Here's how the part is built. I have some questions about the finished solid (model axes, mm). Face numbers are marked on the shaded views. A direction names the side the tool comes from. Give positions to 0.01 mm unless a question says otherwise; leave off trailing zeros. Order: outer loops, then holes, each group sorted by start corner. A loop starts at its lowest first (then second) coordinate and runs counter-clockwise, first axis right, second up. Notation, with made-up numbers: M 43,75.5 L 90,75.5 A6 ccw 90,84.5 Z; hole C 86.5,-4.5 d3. An arc over 180 degrees is marked long. One line per item, written item: value. Start each with the question number.
from build123d import *

# Parameters (mm, degrees)
F0_W          = 62
F0_H          = 90
F1_DEPTH      = 3
F2_W          = 62
F2_H          = 26
F3_DEPTH      = 10
F4_R          = 9.5
F5_DEPTH      = 29
F6_R          = 6
F7_DEPTH      = 31.001
F7_DEPTH_BACK = 31.001
F8_R          = 12.5
F8_R_2        = 1.55
F9_DEPTH      = 13.001
F18_DEPTH     = 2
F19_W         = 8
F19_H         = 25.5
F20_DEPTH     = 10
F21_W         = 8
F21_H         = 2.25
F22_DEPTH     = 10
F23_W         = 8
F23_H         = 4
F24_DEPTH     = 10
F25_SIZE      = 1


with BuildPart() as f1:
    # F0 (on Top) → F1 (new body)
    with BuildSketch(Plane.XY):
        Rectangle(F0_W, F0_H)
    extrude(amount=F1_DEPTH)

    # F2 (on face) → F3 (join)
    with BuildSketch(Plane(origin=(0, 0, 0), x_dir=(1, 0, 0), z_dir=(0, 0, -1))):
        with Locations((0, 32)):
            Rectangle(F2_W, F2_H)
        with Locations((0, -32)):
            Rectangle(F2_W, F2_H)
    extrude(amount=F3_DEPTH)

    # F4 (on Right) → F5 (cut, symmetric)
    with BuildSketch(Plane.YZ):
        with Locations((-32, -10)):
            Circle(F4_R)
        with Locations((32, -10)):
            Circle(F4_R)
    extrude(amount=F5_DEPTH, both=True, mode=Mode.SUBTRACT)

    # F6 (on Right) → F7 (cut, two sides)
    with BuildSketch(Plane.YZ) as f7_sk:
        with Locations((-32, -10)):
            Circle(F6_R)
        with Locations((32, -10)):
            Circle(F6_R)
    extrude(amount=-F7_DEPTH, mode=Mode.SUBTRACT)
    extrude(f7_sk.sketch, amount=F7_DEPTH_BACK, mode=Mode.SUBTRACT)

    # F8 (on face) → F9 (cut, through all)
    with BuildSketch(Plane.XY.offset(3)):
        with Locations((0, -7)):
            Circle(F8_R)
        with Locations((-17.5, -7)):
            Circle(F8_R_2)
        with Locations((17.5, -7)):
            Circle(F8_R_2)
    extrude(amount=-F9_DEPTH, mode=Mode.SUBTRACT)

    # F11 (on offset) + F13 (on offset) + F15 (on offset) + F17 (on offset) → F18 (cut, symmetric)
    with BuildSketch(Plane.YZ.offset(23)):
        with BuildLine():
            Line((-44, 3), (-44, -10))
            Line((-44, -10), (-42, -10))
            Line((-42, -10), (-42, -4))
            ThreePointArc((-42, -4), (-40.5355339059, -0.4644660941), (-37, 1))
            Line((-37, 1), (-27, 1))
            ThreePointArc((-27, 1), (-23.4644660941, -0.4644660941), (-22, -4))
            Line((-22, -4), (-22, -10))
            Line((-22, -10), (-20, -10))
            Line((-20, -10), (-20, 3))
            Line((-20, 3), (-44, 3))
        make_face()
        with BuildLine():
            Line((42, -4), (42, -10))
            Line((42, -10), (44, -10))
            Line((44, -10), (44, 3))
            Line((44, 3), (20, 3))
            Line((20, 3), (20, -10))
            Line((20, -10), (22, -10))
            Line((22, -10), (22, -4))
            ThreePointArc((22, -4), (23.4644660941, -0.4644660941), (27, 1))
            Line((27, 1), (37, 1))
            ThreePointArc((37, 1), (40.5355339059, -0.4644660941), (42, -4))
        make_face()
    with BuildSketch(Plane.YZ.offset(6)):
        with BuildLine():
            Line((-44, 3), (-44, -10))
            Line((-44, -10), (-42, -10))
            Line((-42, -10), (-42, -4))
            ThreePointArc((-42, -4), (-40.5355339059, -0.4644660941), (-37, 1))
            Line((-37, 1), (-27, 1))
            ThreePointArc((-27, 1), (-23.4644660941, -0.4644660941), (-22, -4))
            Line((-22, -4), (-22, -10))
            Line((-22, -10), (-20, -10))
            Line((-20, -10), (-20, 3))
            Line((-20, 3), (-44, 3))
        make_face()
        with BuildLine():
            Line((20, -10), (22, -10))
            Line((22, -10), (22, -4))
            ThreePointArc((22, -4), (23.4644660941, -0.4644660941), (27, 1))
            Line((27, 1), (37, 1))
            ThreePointArc((37, 1), (40.5355339059, -0.4644660941), (42, -4))
            Line((42, -4), (42, -10))
            Line((42, -10), (44, -10))
            Line((44, -10), (44, 3))
            Line((44, 3), (20, 3))
            Line((20, 3), (20, -10))
        make_face()
    with BuildSketch(Plane.YZ.offset(-23)):
        with BuildLine():
            Line((-44, 3), (-44, -10))
            Line((-44, -10), (-42, -10))
            Line((-42, -10), (-42, -4))
            ThreePointArc((-42, -4), (-40.5355339059, -0.4644660941), (-37, 1))
            Line((-37, 1), (-27, 1))
            ThreePointArc((-27, 1), (-23.4644660941, -0.4644660941), (-22, -4))
            Line((-22, -4), (-22, -10))
            Line((-22, -10), (-20, -10))
            Line((-20, -10), (-20, 3))
            Line((-20, 3), (-44, 3))
        make_face()
        with BuildLine():
            Line((42, -10), (44, -10))
            Line((44, -10), (44, 3))
            Line((44, 3), (20, 3))
            Line((20, 3), (20, -10))
            Line((20, -10), (22, -10))
            Line((22, -10), (22, -4))
            ThreePointArc((22, -4), (23.4644660941, -0.4644660941), (27, 1))
            Line((27, 1), (37, 1))
            ThreePointArc((37, 1), (40.5355339059, -0.4644660941), (42, -4))
            Line((42, -4), (42, -10))
        make_face()
    with BuildSketch(Plane.YZ.offset(-6)):
        with BuildLine():
            Line((-44, 3), (-44, -10))
            Line((-44, -10), (-42, -10))
            Line((-42, -10), (-42, -4))
            ThreePointArc((-42, -4), (-40.5355339059, -0.4644660941), (-37, 1))
            Line((-37, 1), (-27, 1))
            ThreePointArc((-27, 1), (-23.4644660941, -0.4644660941), (-22, -4))
            Line((-22, -4), (-22, -10))
            Line((-22, -10), (-20, -10))
            Line((-20, -10), (-20, 3))
            Line((-20, 3), (-44, 3))
        make_face()
        with BuildLine():
            Line((42, -4), (42, -10))
            Line((42, -10), (44, -10))
            Line((44, -10), (44, 3))
            Line((44, 3), (20, 3))
            Line((20, 3), (20, -10))
            Line((20, -10), (22, -10))
            Line((22, -10), (22, -4))
            ThreePointArc((22, -4), (23.4644660941, -0.4644660941), (27, 1))
            Line((27, 1), (37, 1))
            ThreePointArc((37, 1), (40.5355339059, -0.4644660941), (42, -4))
        make_face()
    extrude(amount=F18_DEPTH, both=True, mode=Mode.SUBTRACT)

    # F19 (on face) → F20 (join)
    with BuildSketch(Plane(origin=(0, 0, 0), x_dir=(1, 0, 0), z_dir=(0, 0, -1))):
        with Locations((27, 0)):
            Rectangle(F19_W, F19_H)
        with Locations((-27, 0)):
            Rectangle(F19_W, F19_H)
    extrude(amount=F20_DEPTH)

    # F21 (on face) → F22 (cut, through all)
    with BuildSketch(Plane(origin=(0, 0, -10), x_dir=(1, 0, 0), z_dir=(0, 0, -1))):
        with Locations((-27, 7.625)):
            Rectangle(F21_W, F21_H)
        with Locations((27, -7.625)):
            Rectangle(F21_W, F21_H)
    extrude(amount=-F22_DEPTH, mode=Mode.SUBTRACT)

    # F23 (on face) → F24 (join)
    with BuildSketch(Plane(origin=(0, 0, -10), x_dir=(1, 0, 0), z_dir=(0, 0, -1))):
        with Locations((-27, -10.75)):
            Rectangle(F23_W, F23_H)
        with Locations((27, 10.75)):
            Rectangle(F23_W, F23_H)
        with Locations((-27, -4.5)):
            Rectangle(F23_W, F23_H)
        with Locations((27, 4.5)):
            Rectangle(F23_W, F23_H)
    extrude(amount=F24_DEPTH)

    # F25
    f25_edges = [f1.edges().sort_by_distance(p)[0] for p in [
        (-23, -8.75, -5),
        (-23, -6.5, -5),
        (-23, 6.5, -15),
        (-23, 8.75, -15),
        (23, 6.5, -5),
        (23, 8.75, -5),
        (23, -6.5, -15),
        (23, -8.75, -15),
    ]]
    chamfer(f25_edges, length=F25_SIZE)


solid = f1.part
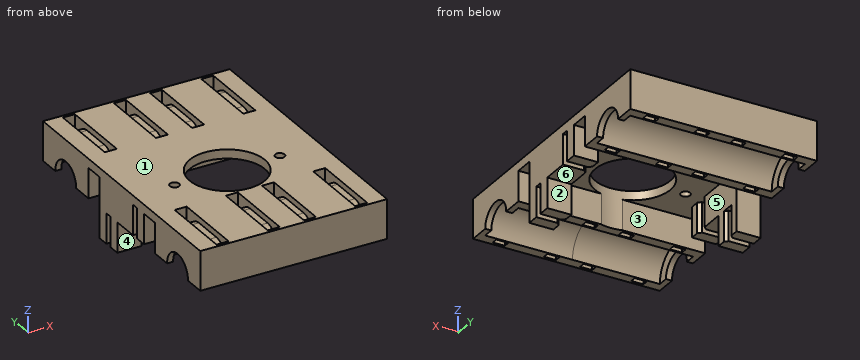
Item 1: Will these pins go through, and if not, where does the flat tip stop? P1, Ø1.5, axis at x = -22, y = 26.5, coming from the -Z side; P2, Ø4, axis at x = 4, y = 17.5, coming from the -Z side; P3, Ø1.2, axis at x = 6, y = -31.5, coming from the +Z side.
Item 2: I want a section at C-C on y = -32. Write out the boundary of the cut face in (x, z), plus the area to 3 significant figures.
Item 3: For the marked faces 4, 5 and 6, which set-ups out of +Z, -Z, +X, -X, +Y, -Y let a thin tool reach every point of the face, with its end or its side?
Item 4: I want a section at A-A on z = -17.5. Write out the boundary of the cut face in (x, y), plus the area to 3 significant figures.
Item 5: I want a section at B-B on x = -17.5. Write out the boundary of the cut face in (y, z), plus the area to 3 significant figures.
Item 6: I want a section at D-D on z = -5.25. Count the separate pieces of the cut face and the enclosed holes in it, plus the area to 3 significant figures.
Item 7: Please list where these lines run through material, in increasing order: probe 1 along X at (y, z) = (40.5, 0.75); probe 2 along X at (y, z) = (11, -1.75); probe 3 along Y at (x, z) = (-13.5, -5.75). Write a range as [from, to].
Item 8: We'd pull the mould along Y, two halves only. Please class the marked faces 1, 2 and 3: +Y half, -Y half, draft (parallel to the pull), parting line (faces both ways), or undercut.
Answer below:
1. P1: stops at z = -2.85
1. P2: stops at z = -10
1. P3: stops at z = 1
2. outline: M -31,-4 L -29,-4 L -29,-0.5 L 29,-0.5 L 29,-4 L 31,-4 L 31,3 L 25,3 L 25,1 L 21,1 L 21,3 L 8,3 L 8,1 L 4,1 L 4,3 L -4,3 L -4,1 L -8,1 L -8,3 L -21,3 L -21,1 L -25,1 L -25,3 L -31,3 Z
2. area: 199 mm²
3. face 4: -Z, +X, -X, -Y
3. face 5: -Z
3. face 6: -Z, +X, +Y
4. outline: M -31,2.5 L -23,2.5 L -23,5.5 L -24,6.5 L -31,6.5 Z; M -31,8.75 L -24,8.75 L -23,9.75 L -23,12.75 L -31,12.75 Z; M 23,-12.75 L 31,-12.75 L 31,-8.75 L 24,-8.75 L 23,-9.75 Z; M 23,-5.5 L 24,-6.5 L 31,-6.5 L 31,-2.5 L 23,-2.5 Z
4. area: 126 mm²
5. outline: M -45,-10 L -41.5,-10 A9.5 cw -22.5,-10 L -19,-10 L -19,0 L -8.55,0 L -8.55,3 L -45,3 Z; M -5.45,0 L 19,0 L 19,-10 L 22.5,-10 A9.5 cw 41.5,-10 L 45,-10 L 45,3 L -5.45,3 Z
5. area: 497 mm²
6. separate pieces: 8
6. enclosed holes: 16
6. area: 1,500 mm²
7. probe 1: x = [-31, -25], [-21, -8], [-4, 4], [8, 21], [25, 31]
7. probe 2: x = [-31, -23], [23, 31]
7. probe 3: y = [-45, -40.5], [-23.5, -19], [19, 23.5], [40.5, 45]
8. face 1: draft
8. face 2: +Y half
8. face 3: undercut
